Input: dimensioned drawing with shaded views. Units: mm. Origin: part minimum x, y, z. A direction names the side the tool comes from. Coordinates: 2 decimals unless noted, no trailing zeros. Order: outer loops, then holes, each group sorted by start corner. A loop starts at its lowest first (then second) coordinate and runs counter-clockwise, first axis right, second up. Notation, with made-up numbers: (39, 19) -> (92, 19) arc R18 ccw to (92, 23) -> close; hole circle Ø6 at (-33, 11.25). An arc over 180 degrees is marked (long way). Answer in a Markdown table with one row per item. Add a question column.
1) Section query B-B on y = 9. Return the cut outline in (x, z).
2) Pull-direction query (Y, two-part tool) for the marked faces 1, 2, 3 and 4; classes: +Y half, -Y half, draft (parallel to the pull), parting line (faces both ways), or undercut.
3) Ray query, line 1 (Y direction, x = 25, z = 3.2); line 2 (Y direction, x = 6.5, z = 3.8) (1 decimal); line 3 (X direction, y = 7.75, z = 2.7). Return the intervals inside material, ascending. Write a range as from..to.
4) Section query A-A on z = 0.75. Count the separate pieces of the cut face and the enclosed holes in it, then the cut area to 3 significant figures.
5) Set-up query: the marked faces 5 and 6. Return all of +Z, -Z, +X, -X, +Y, -Y with unobstructed straight access to the full face (end or side cutting, diameter ignored); none if empty.
6) Section query C-C on x = 13. Return the cut outline in (y, z).
7) Contact query for flat-ended pins moving along their axis: P1, Ø5, axis at x = 25, y = 10, coming from the -Z side; P2, Ø1, axis at y = 3, z = 2, coming from the +X side. Output: stop coordinate, or through.
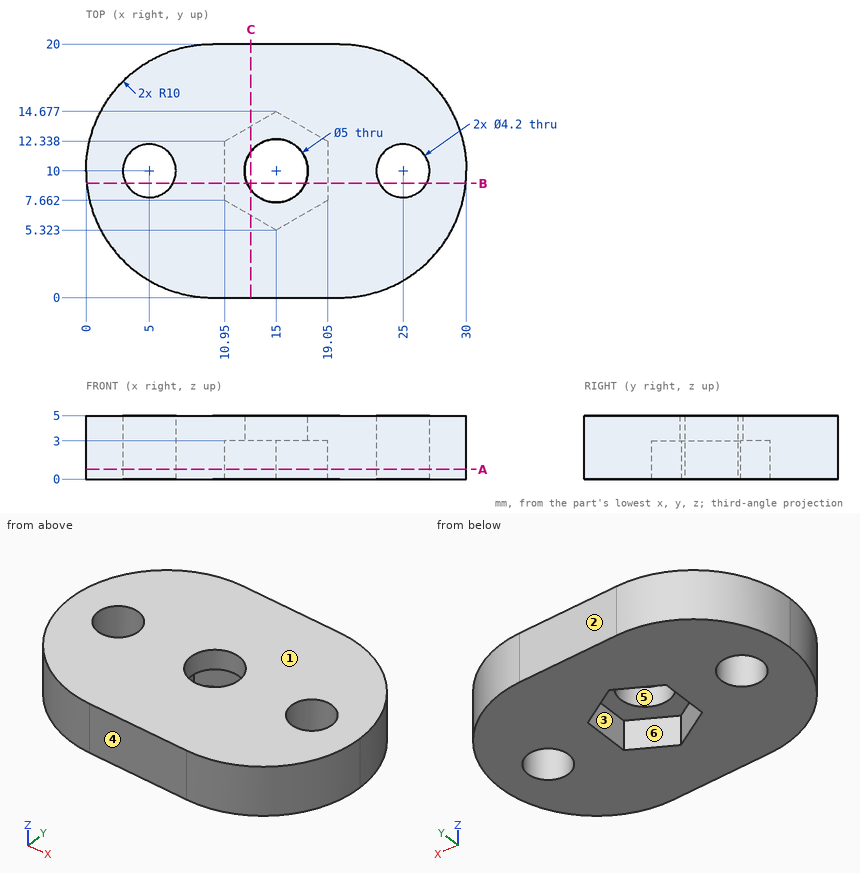
Result:
| question | item | result |
|---|---|---|
| 1 | outline | (0.05, 0) -> (3.15, 0) -> (3.15, 5) -> (0.05, 5) -> close; (6.85, 0) -> (10.95, 0) -> (10.95, 3) -> (12.71, 3) -> (12.71, 5) -> (6.85, 5) -> close; (17.29, 3) -> (19.05, 3) -> (19.05, 0) -> (23.15, 0) -> (23.15, 5) -> (17.29, 5) -> close; (26.85, 0) -> (29.95, 0) -> (29.95, 5) -> (26.85, 5) -> close |
| 2 | face 1 | draft |
| 2 | face 2 | +Y half |
| 2 | face 3 | undercut |
| 2 | face 4 | -Y half |
| 3 | line 1 | 1.34..7.9, 12.1..18.66 |
| 3 | line 2 | 0.6..8.5, 11.5..19.4 |
| 3 | line 3 | 0.26..10.95, 19.05..29.74 |
| 4 | separate pieces | 1 |
| 4 | enclosed holes | 3 |
| 4 | area | 430 mm2 |
| 5 | face 5 | +Z, -Z |
| 5 | face 6 | -Z |
| 6 | outline | (0, 0) -> (6.48, 0) -> (6.48, 3) -> (8.5, 3) -> (8.5, 5) -> (0, 5) -> close; (11.5, 3) -> (13.52, 3) -> (13.52, 0) -> (20, 0) -> (20, 5) -> (11.5, 5) -> close |
| 7 | P1 | z = 0 |
| 7 | P2 | x = 27.6 |
